```python
from build123d import *

# Parameters (mm, degrees)
SKETCH1_W           = 146.4
SKETCH1_H           = 95.25
BOSS_EXTRUDE1_DEPTH = 3
SKETCH2_W           = 6
SKETCH2_H           = 12.7
BOSS_EXTRUDE2_DEPTH = 6
SKETCH3_W           = 12.319
SKETCH3_H           = 6
CUT_EXTRUDE1_DEPTH  = 93.610909859
LPATTERN3_COUNT     = 3
LPATTERN3_PITCH     = 25.4
LPATTERN3_COL_COUNT = 3
LPATTERN3_COL_PITCH = 25.4
CUT_EXTRUDE2_DEPTH  = 93.610909859
FILLET1_R           = 3.175
FILLET2_R           = 1.905


with BuildPart() as part:
    # Sketch1 → Boss-Extrude1 (new, symmetric)
    with BuildSketch(Plane(origin=(0, 0, 0), x_dir=(1, 0, 0), z_dir=(0, 1, 0))):
        Rectangle(SKETCH1_W, SKETCH1_H)
    extrude(amount=BOSS_EXTRUDE1_DEPTH, both=True)

    # Sketch2 → Boss-Extrude2 (add)
    with BuildSketch(Plane(origin=(0, 3, 0), x_dir=(1, 0, 0), z_dir=(0, 1, 0))):
        with Locations((-76.2, 38.1)):
            Rectangle(SKETCH2_W, SKETCH2_H)
        with Locations((-76.2, -38.1)):
            Rectangle(SKETCH2_W, SKETCH2_H)
    boss_extrude2 = extrude(amount=-BOSS_EXTRUDE2_DEPTH)

    # Mirror1: Boss-Extrude2 across plane
    add(boss_extrude2.mirror(Plane(origin=(0, 0, 0), x_dir=(0, 0, 1), z_dir=(1, 0, 0))))

    # Sketch3 → Cut-Extrude1 (cut, symmetric)
    with BuildSketch(Plane(origin=(0, 3, 0), x_dir=(1, 0, 0), z_dir=(0, 1, 0))):
        with Locations((0, 40.005)):
            Rectangle(SKETCH3_W, SKETCH3_H)
        with Locations((0, -40.005)):
            Rectangle(SKETCH3_W, SKETCH3_H)
    cut_extrude1 = extrude(amount=CUT_EXTRUDE1_DEPTH, both=True, mode=Mode.SUBTRACT)

    # LPattern3: Cut-Extrude1 ×3
    with Locations(*[(i * LPATTERN3_PITCH, 0, 0) for i in range(1, LPATTERN3_COUNT)]):
        add(cut_extrude1, mode=Mode.SUBTRACT)

    # LPattern3 col: Cut-Extrude1 ×3
    with Locations(*[(-i * LPATTERN3_COL_PITCH, 0, 0) for i in range(1, LPATTERN3_COL_COUNT)]):
        add(cut_extrude1, mode=Mode.SUBTRACT)

    # Sketch4 → Cut-Extrude2 (cut, through all)
    with BuildSketch(Plane(origin=(0, 3, 0), x_dir=(1, 0, 0), z_dir=(0, 1, 0))):
        Polygon((-7.617051812, 0), (-66.85, 27.16209464), (-66.85, -27.16209464), align=None)
        Polygon((-3.175, 4.948845898), (-3.175, 30.655), (-59.232948188, 30.655), align=None)
        Polygon((59.232948188, 30.655), (3.175, 30.655), (3.175, 4.948845898), align=None)
        Polygon((66.85, -27.16209464), (66.85, 27.16209464), (7.617051812, 0), align=None)
        Polygon((59.232948188, -30.655), (3.175, -4.948845898), (3.175, -30.655), align=None)
        Polygon((-3.175, -30.655), (-3.175, -4.948845898), (-59.232948188, -30.655), align=None)
    extrude(amount=-CUT_EXTRUDE2_DEPTH, mode=Mode.SUBTRACT)

    # Fillet1
    fillet1_edges = [part.edges().sort_by_distance(p)[0] for p in [
        (66.85, 0, -27.16209464),
        (66.85, 0, 27.16209464),
        (7.617051812, 0, 0),
        (3.175, 0, 4.948845898),
        (59.232948188, 0, 30.655),
        (3.175, 0, 30.655),
        (3.175, 0, -30.655),
        (59.232948188, 0, -30.655),
        (3.175, 0, -4.948845898),
        (-59.232948188, 0, -30.655),
        (-3.175, 0, -30.655),
        (-3.175, 0, -4.948845898),
        (-3.175, 0, 4.948845898),
        (-3.175, 0, 30.655),
        (-59.232948188, 0, 30.655),
        (-7.617051812, 0, 0),
        (-66.85, 0, 27.16209464),
        (-66.85, 0, -27.16209464),
    ]]
    fillet(fillet1_edges, radius=FILLET1_R)

    # Fillet2
    fillet2_edges = [part.edges().sort_by_distance(p)[0] for p in [
        (-79.2, 0, -31.75),
        (-79.2, 0, -44.45),
        (-79.2, 0, 44.45),
        (-79.2, 0, 31.75),
        (79.2, 0, -31.75),
        (79.2, 0, -44.45),
        (79.2, 0, 44.45),
        (79.2, 0, 31.75),
        (-73.2, 0, -47.625),
        (73.2, 0, -47.625),
        (73.2, 0, 47.625),
        (-73.2, 0, 47.625),
    ]]
    fillet(fillet2_edges, radius=FILLET2_R)


solid = part.part
```
Can you work these out from the model? Positions are in its coordinate system, mm. A direction names the side the tool comes from. Coordinates: 2 decimals unless noted, no trailing zeros. Order: outer loops, then holes, each group sorted by start corner. A loop starts at its lowest first (then second) coordinate and runs counter-clockwise, first axis right, second up. Notation, with made-up numbers: (65, 59) - (91, 59) arc R24 cw to (91, 71) - close; hole circle Ø10 at (-23, 41). An arc over 180 degrees is marked (long way). Answer in a Markdown table with one row per item.
1. Suppose I cut it at D-D (x = 23.5). Please give me the cut outline in (y, z) (3 decimals), and give its area (3 significant figures).
Reply:
| item | result |
|---|---|
| outline | (-3, -47.625) - (3, -47.625) - (3, -43.005) - (-3, -43.005) - close; (-3, -37.005) - (3, -37.005) - (3, -30.655) - (-3, -30.655) - close; (-3, -14.269) - (3, -14.269) - (3, -7.283) - (-3, -7.283) - close; (-3, 7.283) - (3, 7.283) - (3, 14.269) - (-3, 14.269) - close; (-3, 30.655) - (3, 30.655) - (3, 37.005) - (-3, 37.005) - close; (-3, 43.005) - (3, 43.005) - (3, 47.625) - (-3, 47.625) - close |
| area | 215 mm^2 |
2. For pin 1 (1.5 mm diameter, centred on y = -1, z = 30.5, fed in from -X); pin 2 (1 mm diameter, centred on y = 2, z = 5, fed in from +X); pin 3 (2 mm diameter, centred on x = 76, y = 1, fed in from -Z), each with a flat end and sliding along its axis, tell me the tip position at first contact or that it passes through.
Reply:
| item | result |
|---|---|
| pin 1 | stops at x = -73.2 |
| pin 2 | stops at x = 73.2 |
| pin 3 | stops at z = -44.45 |
3. For faces 1 (the flat face through (-56.96, 0, 40)), 2 (the flat face through (-75, 0, -31.75)), 3 (the flat face through (73.2, 0, 0)), which set-ups out of +Z, -Z, +X, -X, +Y, -Y let a thin tool reach every point of the face, with its end or its side?
Reply:
| item | result |
|---|---|
| face 1 | +Y, -Y |
| face 2 | -X, +Y, -Y |
| face 3 | +X, +Y, -Y |
4. Suppose I cut it at A-A (z = -39.5). Please give me the cut outline in (x, y).
Reply:
| item | result |
|---|---|
| outline | (-79.2, -3) - (-56.96, -3) - (-56.96, 3) - (-79.2, 3) - close; (-44.64, -3) - (-31.56, -3) - (-31.56, 3) - (-44.64, 3) - close; (-19.24, -3) - (-6.16, -3) - (-6.16, 3) - (-19.24, 3) - close; (6.16, -3) - (19.24, -3) - (19.24, 3) - (6.16, 3) - close; (31.56, -3) - (44.64, -3) - (44.64, 3) - (31.56, 3) - close; (56.96, -3) - (79.2, -3) - (79.2, 3) - (56.96, 3) - close |
5. Suppose I cut it at B-B (z = 29). Please give me the cut outline in (x, y).
Reply:
| item | result |
|---|---|
| outline | (-73.2, -3) - (-47.48, -3) - (-47.48, 3) - (-73.2, 3) - close; (-3.56, -3) - (3.56, -3) - (3.56, 3) - (-3.56, 3) - close; (47.48, -3) - (73.2, -3) - (73.2, 3) - (47.48, 3) - close |
6. Suppose I cut it at C-C (y = 0.25). Give the number of separate pieces and of enclosed holes in the cut face, and give its area (3 significant figures).
Reply:
| item | result |
|---|---|
| separate pieces | 1 |
| enclosed holes | 16 |
| area | 7,610 mm^2 |
7. If I drill on line 1 along X through (y, z) = (-0.75, -40.5); line 2 along Z through (x, y) = (-10.5, -2.5) (3 decimals); line 3 along X through (y, z) = (-1.75, -23) (3 decimals), over which ranges is the centre line in solid material (lowest first)?
Reply:
| item | result |
|---|---|
| line 1 | x = -79.2 to -56.96, -44.64 to -31.56, -19.24 to -6.16, 6.16 to 19.24, 31.56 to 44.64, 56.96 to 79.2 |
| line 2 | z = -47.625 to -30.655, -8.308 to 8.308, 30.655 to 47.625 |
| line 3 | x = -73.2 to -66.751, -57.774 to -42.54, -3.175 to 3.175, 42.54 to 57.774, 66.751 to 73.2 |
